from build123d import *

# Parameters (mm, degrees)
SKETCH_1_R          = 37.8
SKETCH_1_R_2        = 26
EXTRUDE_1_DEPTH     = 7
SKETCH_2_R          = 29
CUT_EXTRUDE_1_DEPTH = 5
FILLET_1_R          = 2
SKETCH_3_R          = 1.7
CUT_EXTRUDE_2_DEPTH = 8
SKETCH_4_R          = 2.9
CUT_EXTRUDE_3_DEPTH = 2.5


with BuildPart() as part:
    # 草图1 → 凸台-拉伸1 (new body)
    with BuildSketch(Plane.XY):
        Circle(SKETCH_1_R)
        Circle(SKETCH_1_R_2, mode=Mode.SUBTRACT)
    extrude(amount=EXTRUDE_1_DEPTH)

    # 草图2 → 切除-拉伸1 (cut)
    with BuildSketch(Plane.XY.offset(7)):
        Circle(SKETCH_2_R)
    extrude(amount=-CUT_EXTRUDE_1_DEPTH, mode=Mode.SUBTRACT)

    # 圆角1
    fillet_1_edges = [part.edges().sort_by_distance(p)[0] for p in [
        (-37.8, 0, 0),
    ]]
    fillet(fillet_1_edges, radius=FILLET_1_R)

    # 草图3 → 切除-拉伸2 (cut)
    with BuildSketch(Plane.XY.offset(7)):
        with Locations((0, -34)):
            Circle(SKETCH_3_R)
        with Locations((-34, 0)):
            Circle(SKETCH_3_R)
        with Locations((0, 34)):
            Circle(SKETCH_3_R)
        with Locations((34, 0)):
            Circle(SKETCH_3_R)
    extrude(amount=-CUT_EXTRUDE_2_DEPTH, mode=Mode.SUBTRACT)

    # 草图4 → 切除-拉伸3 (cut)
    with BuildSketch(Plane(origin=(0, 0, 0), x_dir=(-1, 0, 0), z_dir=(0, 0, -1))):
        with Locations((-34, 0)):
            Circle(SKETCH_4_R)
        with Locations((0, 34)):
            Circle(SKETCH_4_R)
        with Locations((34, 0)):
            Circle(SKETCH_4_R)
        with Locations((0, -34)):
            Circle(SKETCH_4_R)
    extrude(amount=-CUT_EXTRUDE_3_DEPTH, mode=Mode.SUBTRACT)


solid = part.part
CAD build for the part. Positions are in the model's coordinates, mm. A direction names the side the tool comes from. Round coordinates to 2 decimals unless told otherwise and drop trailing zeros. Loops run counter-clockwise (first coordinate to the right, second up) from the corner with the lowest first, then second, coordinate; pieces in that order, holes last.
(1) Drop flat-ended pins along their axis: pin 1 (3 mm diameter, centred on x = 7, z = 6, fed in from +Y); pin 2 (4.5 mm diameter, centred on x = 34, y = 0, fed in from +Z); pin 3 (5 mm diameter, centred on x = 0, y = -34, fed in from -Z); pin 4 (1.5 mm diameter, centred on x = -12, z = 6, fed in from +Y). Give the stop position or say it passes through.
(2) Which spindle directions (+Z, -Z, +X, -X, +Y, -Y) get a long thin tool onto all of the face, cutting with end or side? Do faces 1 (the flat face through (-0.2, -26.3, 0)), 2 (the flat face through (-2, 34, 2.5)), 3 (the flat face through (-11, 24, 2)). Say none if no direction does.
(3) Cut at A-A (x = 0). Give the cut face in (y, z).
(4) Two-plate mould, pull along X, no slides. Class faces 4 (the cylindrical face through (-32.38, 0.51, 4.78)), 5 (the cylindrical face through (36.054, 11.354, 4.465)), 6 (the flat face through (-9, -28, 7)): +X half, -X half, draft (parallel to the pull), parting line (faces both ways), or undercut.
(5) Wall check: line 1 along Y through (x, z) = (0, 4.5); line 2 along Y through (x, z) = (32.5, 1.75); line 3 along Y through (x, z) = (-20.5, 6). Give the ranges that are in metal, low to high.
Findings below:
1. pin 1: stops at y = 37.4
1. pin 2: stops at z = 7
1. pin 3: stops at z = 2.5
1. pin 4: stops at y = 36.09
2. face 1: -Z, +X, -X, +Y, -Y
2. face 2: -Z
2. face 3: +Z
3. outline: (-37.8, 2) arc R2 ccw to (-36.9, 0.33) - (-36.9, 2.5) - (-35.7, 2.5) - (-35.7, 7) - (-37.8, 7) - close; (-32.3, 2.5) - (-31.1, 2.5) - (-31.1, 0) - (-26, 0) - (-26, 2) - (-29, 2) - (-29, 7) - (-32.3, 7) - close; (26, 0) - (31.1, 0) - (31.1, 2.5) - (32.3, 2.5) - (32.3, 7) - (29, 7) - (29, 2) - (26, 2) - close; (35.7, 2.5) - (36.9, 2.5) - (36.9, 0.33) arc R2 ccw to (37.8, 2) - (37.8, 7) - (35.7, 7) - close
4. face 4: undercut
4. face 5: parting line
4. face 6: draft
5. line 1: y = -37.8 to -35.7, -32.3 to -29, 29 to 32.3, 35.7 to 37.8
5. line 2: y = -19.27 to -2.48, 2.48 to 19.27
5. line 3: y = -31.76 to -20.51, 20.51 to 31.76
